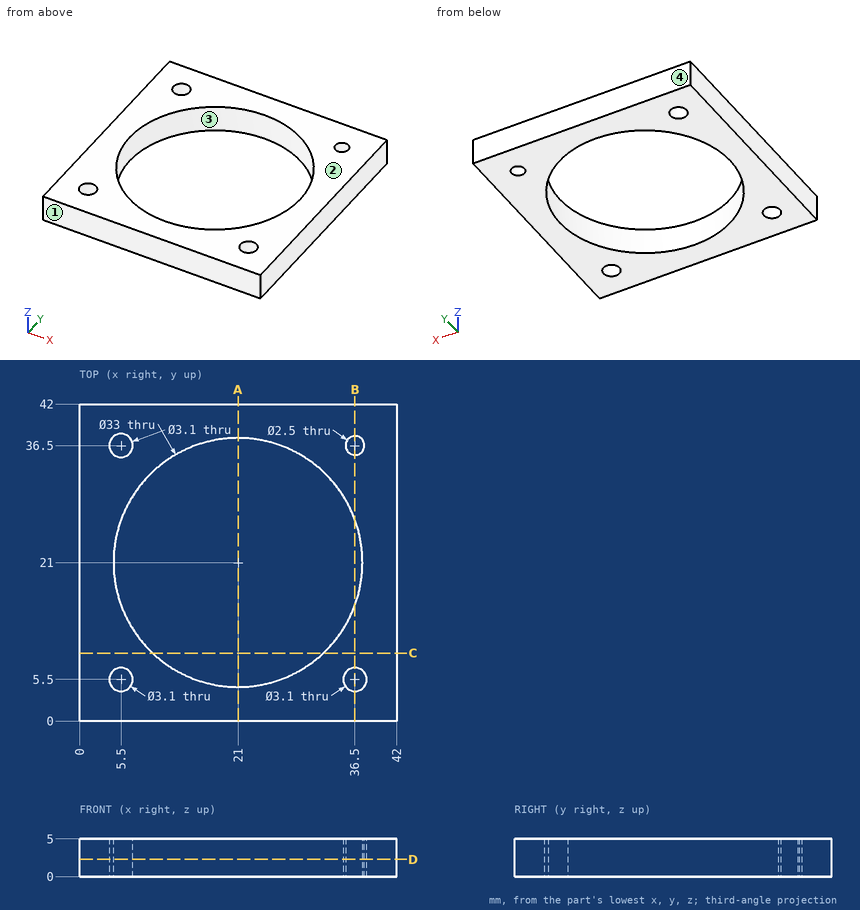
Verification items for this drawing (mm, ordinates from the low corner). Give positions to 0.01 mm unless a question says otherwise; leave off trailing zeros. Loops run counter-clockwise (first coordinate to the right, second up) from the corner with the lowest first, then second, coordinate; pieces in that order, holes last. Notation, with made-up numbers: M -13,44.25 L 9,44.25 A24 ccw 9,74.25 Z; hole C -38,0 d8. An arc over 180 degrees is marked long. Answer in a Markdown table with one row per item.
1) Mould release check, pull along Y, two halves, no side actions. Record for the marked faces 1, 2, 3 and 4: released by +Y, released by -Y, zero draft, split by the parting line, or undercut.
Solutions:
| item | result |
|---|---|
| face 1 | released by -Y |
| face 2 | zero draft |
| face 3 | undercut |
| face 4 | released by +Y |
2) Cross-section at C-C (y = 9). Enter the section's corners in (x, z), plus the area to 3 significant figures.
Solutions:
| item | result |
|---|---|
| outline | M 0,0 L 9.68,0 L 9.68,5 L 0,5 Z; M 32.32,0 L 42,0 L 42,5 L 32.32,5 Z |
| area | 96.8 mm^2 |
3) Cross-section at A-A (x = 21). Enter the section's corners in (y, z), plus the area to 3 significant figures.
Solutions:
| item | result |
|---|---|
| outline | M 0,0 L 4.5,0 L 4.5,5 L 0,5 Z; M 37.5,0 L 42,0 L 42,5 L 37.5,5 Z |
| area | 45.0 mm^2 |
4) Thickness scan on line 1 (X direction, y = 6, z = 1.65); line 2 (Y direction, x = 21, z = 3); line 3 (X direction, y = 31, z = 3.1). Record the ranges inside material, lowest first.
Solutions:
| item | result |
|---|---|
| line 1 | x = 0 to 4.03, 6.97 to 14.13, 27.87 to 35.03, 37.97 to 42 |
| line 2 | y = 0 to 4.5, 37.5 to 42 |
| line 3 | x = 0 to 7.88, 34.12 to 42 |
5) Cross-section at D-D (z = 2.3). Enter the section's corners in (x, y), plus the area to 3 significant figures.
Solutions:
| item | result |
|---|---|
| outline | M 0,0 L 42,0 L 42,42 L 0,42 Z; hole C 5.5,5.5 d3.1; hole C 5.5,36.5 d3.1; hole C 21,21 d33; hole C 36.5,5.5 d3.1; hole C 36.5,36.5 d2.5 |
| area | 881 mm^2 |
6) Cross-section at B-B (x = 36.5). Enter the section's corners in (y, z).
Solutions:
| item | result |
|---|---|
| outline | M 0,0 L 3.95,0 L 3.95,5 L 0,5 Z; M 7.05,0 L 15.34,0 L 15.34,5 L 7.05,5 Z; M 26.66,0 L 35.25,0 L 35.25,5 L 26.66,5 Z; M 37.75,0 L 42,0 L 42,5 L 37.75,5 Z |
